For this review, take the finished solid that the model builds, in its own axes (mm). Face numbers are marked on the shaded views. A direction names the side the tool comes from. Coordinates: 2 decimals unless noted, no trailing zeros. Write each loop counter-clockwise with the first axis right and the second up, starting at its lowest first coordinate (ties: lowest second). Pieces come first, ordered by that corner, then holes.
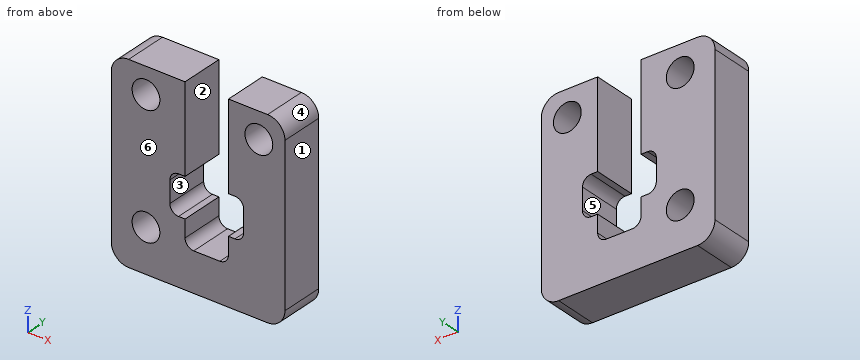
```python
from build123d import *

# Parameters (mm, degrees)
SKETCH_2_W          = 20
SKETCH_2_H          = 22
SKETCH_2_R          = 1.6
SKETCH_2_W_2        = 8.5
SKETCH_2_H_2        = 4.5
EXTRUDE_1_DEPTH     = 5
SKETCH_3_W          = 5
SKETCH_3_H          = 17.5
CUT_EXTRUDE_1_DEPTH = 17.401219467
FILLET_1_R          = 2
FILLET_2_R          = 1


with BuildPart() as part:
    # 草图2 → 凸台-拉伸1 (new body)
    with BuildSketch(Plane(origin=(0, 0, 0), x_dir=(1, 0, 0), z_dir=(0, 1, 0))):
        with Locations((0, 1)):
            Rectangle(SKETCH_2_W, SKETCH_2_H)
        with Locations(Location((-6, -7, 0), (0, 0, 270))):
            Circle(SKETCH_2_R, mode=Mode.SUBTRACT)
        with Locations(Location((7, -7, 0), (0, 0, 270))):
            Circle(SKETCH_2_R, mode=Mode.SUBTRACT)
        with Locations(Location((-6, 7, 0), (0, 0, 270))):
            Circle(SKETCH_2_R, mode=Mode.SUBTRACT)
        with Locations((1, 2.25)):
            Rectangle(SKETCH_2_W_2, SKETCH_2_H_2, mode=Mode.SUBTRACT)
    extrude(amount=EXTRUDE_1_DEPTH)

    # 草图3 → 切除-拉伸1 (cut, through all)
    with BuildSketch(Plane.XZ):
        with Locations((1, 1.25)):
            Rectangle(SKETCH_3_W, SKETCH_3_H)
    extrude(amount=-CUT_EXTRUDE_1_DEPTH, mode=Mode.SUBTRACT)

    # 圆角1
    fillet_1_edges = [part.edges().sort_by_distance(p)[0] for p in [
        (10, 2.5, 10),
        (-10, 2.5, 10),
        (-10, 2.5, -12),
        (10, 2.5, -12),
    ]]
    fillet(fillet_1_edges, radius=FILLET_1_R)

    # 圆角2
    fillet_2_edges = [part.edges().sort_by_distance(p)[0] for p in [
        (5.25, 2.5, -4.5),
        (-3.25, 2.5, -4.5),
        (-3.25, 2.5, 0),
        (5.25, 2.5, 0),
        (-1.5, 2.5, -7.5),
        (3.5, 2.5, -7.5),
    ]]
    fillet(fillet_2_edges, radius=FILLET_2_R)


solid = part.part
```
Q1. Add section A-A (z = 7). State the section outline as (x, y) points.
Ans:
outline: (-10, 0) - (-7.6, 0) - (-7.6, 5) - (-10, 5) - close; (-4.4, 0) - (-1.5, 0) - (-1.5, 5) - (-4.4, 5) - close; (3.5, 0) - (5.4, 0) - (5.4, 5) - (3.5, 5) - close; (8.6, 0) - (10, 0) - (10, 5) - (8.6, 5) - close
Q2. Draft analysis for pull direction Z (two halves, no side actions). For the marked faces 4, 5 and 6, state which applies: +Z half, -Z half, draft (parallel to the pull), parting line (faces both ways), or undercut.
Ans:
face 4: +Z half
face 5: undercut
face 6: draft
Q3. Add section C-C (y = 1.1). Give the number of separate pieces and of enclosed holes in the cut face, then the cut area to 3 significant figures.
Ans:
separate pieces: 1
enclosed holes: 3
area: 310 mm2
Q4. Add section B-B (x = -6). State the section outline as (y, z) points.
Ans:
outline: (0, -12) - (5, -12) - (5, -8.6) - (0, -8.6) - close; (0, -5.4) - (5, -5.4) - (5, 5.4) - (0, 5.4) - close; (0, 8.6) - (5, 8.6) - (5, 10) - (0, 10) - close
Q5. Add section D-D (z = 1.5). State the section outline as (x, y) points.
Ans:
outline: (-10, 0) - (-1.5, 0) - (-1.5, 5) - (-10, 5) - close; (3.5, 0) - (10, 0) - (10, 5) - (3.5, 5) - close
Q6. Clearance check with a flat-ended pin moving along its axis: pin 1 Ø1.5 at (x, y) = (1, 2.5) entering from +Z. State where the tip first meets the part, or that it passes through.
Ans:
pin 1: stops at z = -7.5
Q7. Tool access review of the marked faces 1, 2 and 3: name each direction out of +Z, -Z, +X, -X, +Y, -Y from which nothing blocks a thin tool from reaching the whole face with its end or side.
Ans:
face 1: +Z, -Z, +X, +Y, -Y
face 2: +Z, +Y, -Y
face 3: +Y, -Y
Q8. For probe 1 along X at (y, z) = (2.6, 7); probe 2 along X at (y, z) = (3.35, -6.5); probe 3 along X at (y, z) = (4.35, 5), list the stretches that pass through material, from the lowest coordinate up.
Ans:
probe 1: x = -10 to -7.6, -4.4 to -1.5, 3.5 to 5.4, 8.6 to 10
probe 2: x = -10 to -7.52, -4.48 to -1.5, 3.5 to 10
probe 3: x = -10 to -1.5, 3.5 to 10
